Here's how the part is built. I have some questions about the finished solid (model axes, mm). A direction names the side the tool comes from. Give positions to 0.01 mm unless a question says otherwise; leave off trailing zeros. Loops run counter-clockwise (first coordinate to the right, second up) from the corner with the lowest first, then second, coordinate; pieces in that order, holes last.
Q1. Thinking about a two-plate mould opening in X: for faces 3 (the face through (0, 0, 0)), 4 (the face through (-0.54, 3.46, -2.44)), which applies, pulls with the +X half, pulls with the -X half, needs draft (parallel to the pull), parting line crosses it, or undercut?
Q2. I'm going to push a flat-ended pin straight in: P1, Ø1, axis at x = -1, z = 2, coming from the -Y side. Where does the tip first touch, or does it pass through?
Q3. Suppose I cut it at A-A (z = 0). List the corners of the cut face in (x, y) for me.
Q4. I need wall thicknesses on probe 1 along X at (y, z) = (4.75, -0.1); probe 2 along X at (y, z) = (2.5, 1.15); probe 3 along Z at (x, y) = (1, 7). Which ranges of each line are inside material? Lowest first, please.
Q5. Suppose I cut it at D-D (y = 4). List the corners of the cut face in (x, z) for me, and give its area (3 significant figures).
Q6. Suppose I cut it at B-B (x = 0). List the corners of the cut face in (y, z) for me.
Q7. For faces 1 (the face through (2, 1, 2)), 2 (the face through (3, 0.5, -0.1)), which set-ups out of +Z, -Z, +X, -X, +Y, -Y let a thin tool reach every point of the face, with its end or its side?
Q8. Suppose I cut it at C-C (y = 7.5). List the corners of the cut face in (x, z) for me, and give its area (3 significant figures).
Autodesk Inventor part; units mm, degrees
ref_plane "YZ Plane" through (0, 0, 0) normal (1, 0, 0) x (0, 1, 0)
ref_plane "XZ Plane" through (0, 0, 0) normal (0, 1, 0) x (-1, 0, 0)
ref_plane "XY Plane" through (0, 0, 0) normal (0, 0, 1) x (1, 0, 0)
sketch "Sketch1" plane through (0, 0, 0) normal (0, 1, 0) x (-1, 0, 0)
  circle A0 centre (0, 0) radius 3
  dimension "d0" = 6
extrude "Extrusion1" add sketch "Sketch1" along normal blind 1
sketch "Sketch2" plane through (0, 1, 0) normal (0, 1, 0) x (1, 0, 0)
  circle A0 centre (0, 0) radius 2.5
  dimension "d3" = 5
extrude "Extrusion2" add sketch "Sketch2" along normal blind 5
sketch "Sketch4" plane through (0, 0, 0) normal (1, 0, 0) x (0, 1, 0)
  line L0 (6, -2.5) -> (6, 2.5)
  line L1 (1, 2.5) -> (1, -2.5)
  line L2 (1, 2.5) -> (6, 2.5)
  line L3 (6, -2.5) -> (6, 2.5)
  arc A0 (8.5, 0) -> (6, 2.5) centre (6, 0) ccw
  line L4 (8.5, 0) -> (6, 0)
  point P0 (0, 0)
revolve "Revolution1" add sketch "Sketch4" angle 360 about axis through (0, 8.5, 0) along (0, -1, 0)
properties part number "LED5mm" material "Glass"
Solutions:
1. face 3: needs draft
1. face 4: parting line crosses it
2. P1: stops at y = 0
3. outline: (-3, 0) - (3, 0) - (3, 1) - (2.5, 1) - (2.5, 6) arc R2.5 ccw to (-2.5, 6) - (-2.5, 1) - (-3, 1) - close
4. probe 1: x = -2.5 to 2.5
4. probe 2: x = -2.22 to 2.22
4. probe 3: z = -2.06 to 2.06
5. outline: circle Ø5 at (0, 0)
5. area: 19.6 mm2
6. outline: (0, -3) - (1, -3) - (1, -2.5) - (6, -2.5) arc R2.5 ccw to (6, 2.5) - (1, 2.5) - (1, 3) - (0, 3) - close
7. face 1: +Y
7. face 2: +Y, -Y
8. outline: circle Ø4 at (0, 0)
8. area: 12.6 mm2
